Geometry: final body of the model. Coordinates: model frame, mm. A direction names the side the tool comes from. Give positions to 0.01 mm unless a question says otherwise; leave off trailing zeros. Write each loop counter-clockwise with the first axis right and the second up, starting at its lowest first coordinate (ties: lowest second). Pieces come first, ordered by that corner, then holes. Notation, with made-up numbers: (27, 75) -> (52, 75) arc R20 cw to (52, 109) -> close; hole circle Ø3 at (66, -21). An arc over 180 degrees is marked (long way). Answer as a JSON object with one key per item and string values. Group by question number.
(1) Section query B-B on z = 18. Output: boundary loops of the cut face in (x, y).
(2) Section query D-D on z = -1. Output: boundary loops of the cut face in (x, y), plus the area to 3 significant figures.
(3) Material intervals for probe 1 along X at (y, z) = (18.25, 2.5); probe 2 along Y at (x, z) = (-1, 18); probe 3 along X at (y, z) = (17.75, -17.5), sorted ascending.
(4) Section query A-A on y = 15. Output: boundary loops of the cut face in (x, z).
(5) Set-up query: faces 1 (the face through (13, 16, 0)), 2 (the face through (21, 16, -8.5)), 3 (the face through (28.4, 16, 15)). Return all of +Z, -Z, +X, -X, +Y, -Y with unobstructed straight access to the full face (end or side cutting, diameter ignored); none if empty.
(6) Section query C-C on x = 3.5. Output: boundary loops of the cut face in (y, z).
(7) Contact query for flat-ended pins moving along their axis: pin 1 Ø6.5 at (x, y) = (20.5, 17) entering from +Z; pin 2 Ø1.8 at (x, y) = (20.5, 16.5) entering from -Z; pin 3 Ø5 at (y, z) = (16.5, 0.5) entering from -X. Output: stop coordinate, or through.
from build123d import *

# Parameters (mm, degrees)
SKETCH_1_W          = 60
SKETCH_1_H          = 44
EXTRUDE_1_DEPTH     = 19
SKETCH_2_W          = 58.4
SKETCH_2_H          = 6
CUT_EXTRUDE_1_DEPTH = 57.542019773
SKETCH_3_W          = 15.4
SKETCH_3_H          = 17
EXTRUDE_2_DEPTH     = 6


with BuildPart() as part:
    # 草图1 → 凸台-拉伸1 (new body)
    with BuildSketch(Plane(origin=(0, 19, 0), x_dir=(1, 0, 0), z_dir=(0, 1, 0))):
        Rectangle(SKETCH_1_W, SKETCH_1_H)
    extrude(amount=-EXTRUDE_1_DEPTH)

    # 草图2 → 切除-拉伸1 (cut, through all)
    with BuildSketch(Plane(origin=(0, 0, -22), x_dir=(-1, 0, 0), z_dir=(0, 0, -1))):
        with Locations((0.8, 16)):
            Rectangle(SKETCH_2_W, SKETCH_2_H)
    extrude(amount=-CUT_EXTRUDE_1_DEPTH, mode=Mode.SUBTRACT)

    # 草图3 → 凸台-拉伸2 (add)
    with BuildSketch(Plane(origin=(0, 13, 0), x_dir=(-1, 0, 0), z_dir=(0, 1, 0))):
        with Locations((-20.7, 0)):
            Rectangle(SKETCH_3_W, SKETCH_3_H)
    extrude(amount=EXTRUDE_2_DEPTH)


solid = part.part
Answer list:
{
 "1": {"outline": "(-30, 0) -> (30, 0) -> (30, 19) -> (28.4, 19) -> (28.4, 13) -> (-30, 13) -> close"},
 "2": {"outline": "(-30, 0) -> (30, 0) -> (30, 19) -> (13, 19) -> (13, 13) -> (-30, 13) -> close", "area": "882 mm2"},
 "3": {"probe 1": "13 to 30", "probe 2": "0 to 13", "probe 3": "28.4 to 30"},
 "4": {"outline": "(13, -8.5) -> (28.4, -8.5) -> (28.4, -22) -> (30, -22) -> (30, 22) -> (28.4, 22) -> (28.4, 8.5) -> (13, 8.5) -> close"},
 "5": {"face 1": "+Z, -Z, -X, +Y", "face 2": "-Z, -X, +Y", "face 3": "+Z, -X, +Y"},
 "6": {"outline": "(0, -22) -> (13, -22) -> (13, 22) -> (0, 22) -> close"},
 "7": {"pin 1": "z = 8.5", "pin 2": "z = -8.5", "pin 3": "x = 13"}
}
